```python
from build123d import *

# Parameters (mm, degrees)
F1_DEPTH = 10
F3_DEPTH = 10.001


with BuildPart() as f1:
    # F0 (on Top) → F1 (new body)
    with BuildSketch(Plane.XY):
        with BuildLine():
            Line((1.950903, 9.807853), (4.389532, 22.067669))
            ThreePointArc((4.389532, 22.067669), (0, 22.5), (-4.389532, 22.067669))
            Line((-4.389532, 22.067669), (-1.950903, 9.807853))
            ThreePointArc((-1.950903, 9.807853), (-2.731096, 9.619829), (-3.493699, 9.369849))
            Line((-3.493699, 9.369849), (-8.733502, 20.735861))
            ThreePointArc((-8.733502, 20.735861), (-9.419844, 20.433221), (-10.095717, 20.107872))
            Line((-10.095717, 20.107872), (-4.855913, 8.741859))
            ThreePointArc((-4.855913, 8.741859), (-5.224986, 8.526402), (-5.584515, 8.295372))
            Line((-5.584515, 8.295372), (-13.332885, 18.124132))
            ThreePointArc((-13.332885, 18.124132), (-13.929614, 17.669631), (-14.510861, 17.195491))
            Line((-14.510861, 17.195491), (-6.762491, 7.366731))
            ThreePointArc((-6.762491, 7.366731), (-7.071068, 7.071068), (-7.366731, 6.762491))
            Line((-7.366731, 6.762491), (-17.195491, 14.510861))
            ThreePointArc((-17.195491, 14.510861), (-17.669631, 13.929614), (-18.124132, 13.332885))
            Line((-18.124132, 13.332885), (-8.295372, 5.584515))
            ThreePointArc((-8.295372, 5.584515), (-8.526402, 5.224986), (-8.741859, 4.855913))
            Line((-8.741859, 4.855913), (-20.107872, 10.095717))
            ThreePointArc((-20.107872, 10.095717), (-20.433221, 9.419844), (-20.735861, 8.733502))
            Line((-20.735861, 8.733502), (-9.369849, 3.493699))
            ThreePointArc((-9.369849, 3.493699), (-9.619829, 2.731096), (-9.807853, 1.950903))
            Line((-9.807853, 1.950903), (-22.067669, 4.389532))
            ThreePointArc((-22.067669, 4.389532), (-22.5, 0), (-22.067669, -4.389532))
            Line((-22.067669, -4.389532), (-9.807853, -1.950903))
            ThreePointArc((-9.807853, -1.950903), (-9.619829, -2.731096), (-9.369849, -3.493699))
            Line((-9.369849, -3.493699), (-20.735861, -8.733502))
            ThreePointArc((-20.735861, -8.733502), (-20.433221, -9.419844), (-20.107872, -10.095717))
            Line((-20.107872, -10.095717), (-8.741859, -4.855913))
            ThreePointArc((-8.741859, -4.855913), (-8.526402, -5.224986), (-8.295372, -5.584515))
            Line((-8.295372, -5.584515), (-18.124132, -13.332885))
            ThreePointArc((-18.124132, -13.332885), (-17.669631, -13.929614), (-17.195491, -14.510861))
            Line((-17.195491, -14.510861), (-7.366731, -6.762491))
            ThreePointArc((-7.366731, -6.762491), (-7.071068, -7.071068), (-6.762491, -7.366731))
            Line((-6.762491, -7.366731), (-14.510861, -17.195491))
            ThreePointArc((-14.510861, -17.195491), (-13.929614, -17.669631), (-13.332885, -18.124132))
            Line((-13.332885, -18.124132), (-5.584515, -8.295372))
            ThreePointArc((-5.584515, -8.295372), (-5.224986, -8.526402), (-4.855913, -8.741859))
            Line((-4.855913, -8.741859), (-10.095717, -20.107872))
            ThreePointArc((-10.095717, -20.107872), (-9.419844, -20.433221), (-8.733502, -20.735861))
            Line((-8.733502, -20.735861), (-3.493699, -9.369849))
            ThreePointArc((-3.493699, -9.369849), (-2.731096, -9.619829), (-1.950903, -9.807853))
            Line((-1.950903, -9.807853), (-4.389532, -22.067669))
            ThreePointArc((-4.389532, -22.067669), (0, -22.5), (4.389532, -22.067669))
            Line((4.389532, -22.067669), (1.950903, -9.807853))
            ThreePointArc((1.950903, -9.807853), (2.731096, -9.619829), (3.493699, -9.369849))
            Line((3.493699, -9.369849), (8.733502, -20.735861))
            ThreePointArc((8.733502, -20.735861), (9.419844, -20.433221), (10.095717, -20.107872))
            Line((10.095717, -20.107872), (4.855913, -8.741859))
            ThreePointArc((4.855913, -8.741859), (5.224986, -8.526402), (5.584515, -8.295372))
            Line((5.584515, -8.295372), (13.332885, -18.124132))
            ThreePointArc((13.332885, -18.124132), (13.929614, -17.669631), (14.510861, -17.195491))
            Line((14.510861, -17.195491), (6.762491, -7.366731))
            ThreePointArc((6.762491, -7.366731), (7.071068, -7.071068), (7.366731, -6.762491))
            Line((7.366731, -6.762491), (17.195491, -14.510861))
            ThreePointArc((17.195491, -14.510861), (17.669631, -13.929614), (18.124132, -13.332885))
            Line((18.124132, -13.332885), (8.295372, -5.584515))
            ThreePointArc((8.295372, -5.584515), (8.526402, -5.224986), (8.741859, -4.855913))
            Line((8.741859, -4.855913), (20.107872, -10.095717))
            ThreePointArc((20.107872, -10.095717), (20.433221, -9.419844), (20.735861, -8.733502))
            Line((20.735861, -8.733502), (9.369849, -3.493699))
            ThreePointArc((9.369849, -3.493699), (9.619829, -2.731096), (9.807853, -1.950903))
            Line((9.807853, -1.950903), (22.067669, -4.389532))
            ThreePointArc((22.067669, -4.389532), (22.5, 0), (22.067669, 4.389532))
            Line((22.067669, 4.389532), (9.807853, 1.950903))
            ThreePointArc((9.807853, 1.950903), (9.619829, 2.731096), (9.369849, 3.493699))
            Line((9.369849, 3.493699), (20.735861, 8.733502))
            ThreePointArc((20.735861, 8.733502), (20.433221, 9.419844), (20.107872, 10.095717))
            Line((20.107872, 10.095717), (8.741859, 4.855913))
            ThreePointArc((8.741859, 4.855913), (8.526402, 5.224986), (8.295372, 5.584515))
            Line((8.295372, 5.584515), (18.124132, 13.332885))
            ThreePointArc((18.124132, 13.332885), (17.669631, 13.929614), (17.195491, 14.510861))
            Line((17.195491, 14.510861), (7.366731, 6.762491))
            ThreePointArc((7.366731, 6.762491), (7.071068, 7.071068), (6.762491, 7.366731))
            Line((6.762491, 7.366731), (14.510861, 17.195491))
            ThreePointArc((14.510861, 17.195491), (13.929614, 17.669631), (13.332885, 18.124132))
            Line((13.332885, 18.124132), (5.584515, 8.295372))
            ThreePointArc((5.584515, 8.295372), (5.224986, 8.526402), (4.855913, 8.741859))
            Line((4.855913, 8.741859), (10.095717, 20.107872))
            ThreePointArc((10.095717, 20.107872), (9.419844, 20.433221), (8.733502, 20.735861))
            Line((8.733502, 20.735861), (3.493699, 9.369849))
            ThreePointArc((3.493699, 9.369849), (2.731096, 9.619829), (1.950903, 9.807853))
        make_face()
    extrude(amount=F1_DEPTH)

    # F2 (on face) → F3 (cut, through all)
    with BuildSketch(Plane.XY.offset(10)):
        with BuildLine():
            Line((22.067669, 4.389532), (9.807853, 1.950903))
            Line((9.807853, 1.950903), (9.807853, -1.950903))
            Line((9.807853, -1.950903), (22.067669, -4.389532))
            ThreePointArc((22.067669, -4.389532), (22.5, 0), (22.067669, 4.389532))
        make_face()
    extrude(amount=-F3_DEPTH, mode=Mode.SUBTRACT)


solid = f1.part
```
Here's how the part is built. I have some questions about the finished solid (model axes, mm). A direction names the side the tool comes from. Give positions to 0.01 mm unless a question says otherwise; leave off trailing zeros. Order: outer loops, then holes, each group sorted by start corner. A loop starts at its lowest first (then second) coordinate and runs counter-clockwise, first axis right, second up. Notation, with made-up numbers: M 21.25,84 L 38.25,84 A18 cw 38.25,99 Z; hole C 6.25,42.25 d10. An arc over 180 degrees is marked long. Use a Markdown table: item, result. Add a question column.
1. Suppose I cut it at C-C (x = 2.5). List the corners of the cut face in (y, z) for me.
2. On a 3-axis mill with a long thin cutter (end or side, diameter ignored), from which of +Z, -Z, +X, -X, +Y, -Y can I reach the whole of each face in a straight line? I mean faces 1 (the flat face through (3.187, -16.024, 4.93)), 2 (the cylindrical face through (-13.94, -17.66, 4.93)), 3 (the cylindrical face through (9.623, 2.72, 4.93)). Say none if no direction works.
3. For pin 1 Ø5 at (y, z) = (1, 4) entering from -X; pin 2 Ø3 at (x, z) = (2, 5) entering from +Y; pin 3 Ø1 at (x, z) = (-11.5, 2) entering from -Y; pin 4 Ø4 at (y, z) = (-5.5, 5) entering from -X, each with a flat end and sliding along its axis, tell me the tip position at first contact or that it passes through.
4. Suppose I cut it at A-A (x = -12). List the corners of the cut face in (y, z) for me (3 decimals), and give its area (3 significant figures).
5. I need wall thicknesses on probe 1 along Y at (x, z) = (17, 3.5); probe 2 along X at (y, z) = (5.5, 7.75); probe 3 along Y at (x, z) = (6, 6.25). Which ranges of each line are inside material? Lowest first, please. Write a range as from..to.
6. Suppose I cut it at D-D (x = 14). List the corners of the cut face in (y, z) for me.
7. If we mould it in two halves opening along Y, with no side actions, what happens to faces 4 (the cylindrical face through (9.617, -2.742, 4.93)), 5 (the flat face through (10.58, 12.21, 4.93)), 6 (the cylindrical face through (9.41, -20.438, 4.93)), 7 (the cylindrical face through (-20.43, 9.43, 4.93))? For each: +Y half, -Y half, draft (parallel to the pull), parting line (faces both ways), or undercut.
8. Suppose I cut it at B-B (y = -14). List the corners of the cut face in (x, z) for me.
Results list:
| question | item | result |
|---|---|---|
| 1 | outline | M -22.36,0 L -12.57,0 L -12.57,10 L -22.36,10 Z; M -9.68,0 L 9.68,0 L 9.68,10 L -9.68,10 Z; M 12.57,0 L 22.36,0 L 22.36,10 L 12.57,10 Z |
| 2 | face 1 | +Z, -Z |
| 2 | face 2 | +Z, -Z, -X, -Y |
| 2 | face 3 | +Z, -Z, +X |
| 3 | pin 1 | stops at x = -22.5 |
| 3 | pin 2 | stops at y = 22.49 |
| 3 | pin 3 | stops at y = -16.43 |
| 3 | pin 4 | stops at x = -22.23 |
| 4 | outline | M -16.433,0 L -14.01,0 L -14.01,10 L -16.433,10 Z; M -10.415,0 L -8.505,0 L -8.505,10 L -10.415,10 Z; M -6.358,0 L -4.706,0 L -4.706,10 L -6.358,10 Z; M -2.387,0 L 2.387,0 L 2.387,10 L -2.387,10 Z; M 4.706,0 L 6.358,0 L 6.358,10 L 4.706,10 Z; M 8.505,0 L 10.415,0 L 10.415,10 L 8.505,10 Z; M 14.01,0 L 16.433,0 L 16.433,10 L 14.01,10 Z |
| 4 | area | 167 mm² |
| 5 | probe 1 | y = -14.36..-12.45, -8.66..-7.01, 7.01..8.66, 12.45..14.36 |
| 5 | probe 2 | x = -13.72..-10.14, -8.35..8.35, 10.14..13.72 |
| 5 | probe 3 | y = -14.81..-11.22, -8.82..8.82, 11.22..14.81 |
| 6 | outline | M -17.61,0 L -16.55,0 L -16.55,10 L -17.61,10 Z; M -11.99,0 L -10.08,0 L -10.08,10 L -11.99,10 Z; M -7.28,0 L -5.63,0 L -5.63,10 L -7.28,10 Z; M 5.63,0 L 7.28,0 L 7.28,10 L 5.63,10 Z; M 10.08,0 L 11.99,0 L 11.99,10 L 10.08,10 Z; M 16.55,0 L 17.61,0 L 17.61,10 L 16.55,10 Z |
| 7 | face 4 | undercut |
| 7 | face 5 | undercut |
| 7 | face 6 | -Y half |
| 7 | face 7 | +Y half |
| 8 | outline | M -17.61,0 L -16.55,0 L -16.55,10 L -17.61,10 Z; M -11.99,0 L -10.08,0 L -10.08,10 L -11.99,10 Z; M -7.28,0 L -5.63,0 L -5.63,10 L -7.28,10 Z; M -2.78,0 L 2.78,0 L 2.78,10 L -2.78,10 Z; M 5.63,0 L 7.28,0 L 7.28,10 L 5.63,10 Z; M 10.08,0 L 11.99,0 L 11.99,10 L 10.08,10 Z; M 16.55,0 L 17.61,0 L 17.61,10 L 16.55,10 Z |
